Could you check a few things on this drawing? It's one solid part, dimensions in mm from its lowest x, y, z. A direction names the side the tool comes from. Round coordinates to 2 decimals unless told otherwise and drop trailing zeros. Write each loop counter-clockwise with the first axis right and the second up, starting at its lowest first coordinate (ties: lowest second). Pieces come first, ordered by that corner, then holes. Notation, with made-up numbers: (59, 42) -> (97, 42) arc R14 cw to (97, 69) -> close; hole circle Ø4 at (5.5, -7.75). An arc over 180 degrees is marked (long way). Answer in a Markdown table with one row per item. Add a question column.
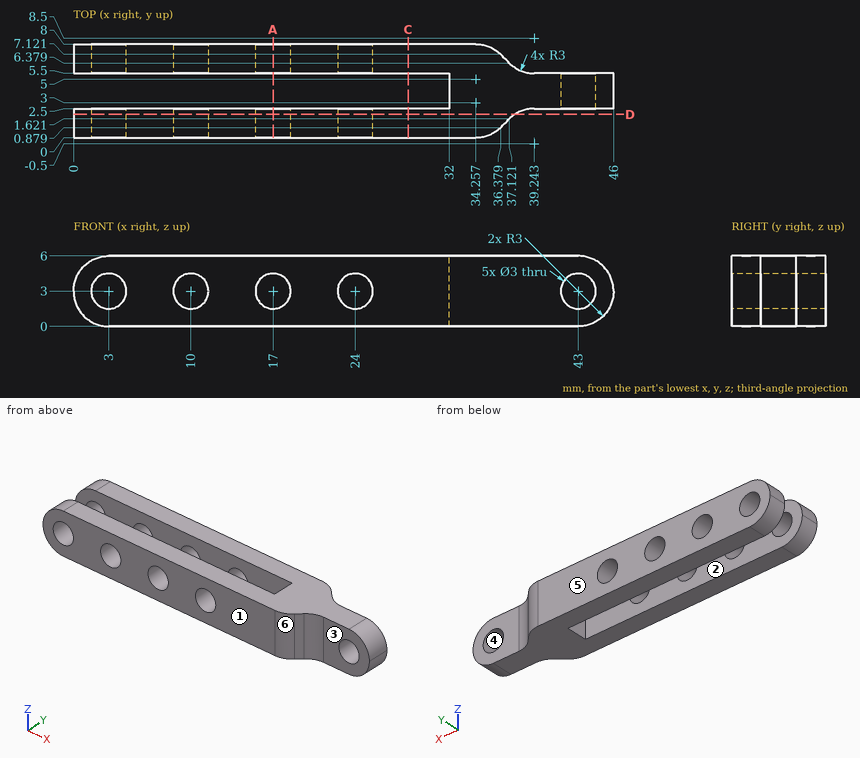
(1) Suppose I cut it at A-A, the plane x = 17. Please give me the cut outline in (y, z).
(2) Suppose I cut it at C-C, the plane x = 28.5. Please give me the cut outline in (y, z).
(3) For P1, Ø3, axis at x = 44.5, z = 3, coming from the -Y side; P2, Ø0.9, axis at y = 4, z = 3, coming from the -X side; P3, Ø1, axis at x = 41, z = 2, coming from the +Y side, each with a flat end and sliding along its axis, tell me the tip position at first contact or that it passes through.
(4) If we mould it in two halves opening along X, with no side actions, what happens to the marked faces 4, 5 and 6? For each: pulls with the +X half, pulls with the -X half, needs draft (parallel to the pull), parting line crosses it, or undercut.
(5) I need wall thicknesses on L1, parallel to Y at x = 2, z = 1; L2, parallel to Z at x = 24, y = 1.7; L3, parallel to X at y = 1.75, z = 2. Which ranges of each line are inside material? Lowest first, please.
(6) Suppose I cut it at D-D, the plane y = 2. State how many separate pieces and enclosed holes the cut face has, then the cut area to 3 significant figures.
(7) On a 3-axis mill with a long thin cutter (end or side, diameter ignored), from which of +Z, -Z, +X, -X, +Y, -Y can I reach the whole of each face in a straight line? I mean the marked faces 1, 2 and 3. Say none if no direction works.
Response:
| question | item | result |
|---|---|---|
| 1 | outline | (0, 0) -> (2.5, 0) -> (2.5, 1.5) -> (0, 1.5) -> close; (0, 4.5) -> (2.5, 4.5) -> (2.5, 6) -> (0, 6) -> close; (5.5, 0) -> (8, 0) -> (8, 1.5) -> (5.5, 1.5) -> close; (5.5, 4.5) -> (8, 4.5) -> (8, 6) -> (5.5, 6) -> close |
| 2 | outline | (0, 0) -> (2.5, 0) -> (2.5, 6) -> (0, 6) -> close; (5.5, 0) -> (8, 0) -> (8, 6) -> (5.5, 6) -> close |
| 3 | P1 | y = 2.5 |
| 3 | P2 | x = 32 |
| 3 | P3 | y = 5.5 |
| 4 | face 4 | undercut |
| 4 | face 5 | needs draft |
| 4 | face 6 | pulls with the +X half |
| 5 | L1 | 0 to 2.5, 5.5 to 8 |
| 5 | L2 | 0 to 1.5, 4.5 to 6 |
| 5 | L3 | 0.17 to 1.88, 4.12 to 8.88, 11.12 to 15.88, 18.12 to 22.88, 25.12 to 37.26 |
| 6 | separate pieces | 1 |
| 6 | enclosed holes | 4 |
| 6 | area | 193 mm² |
| 7 | face 1 | +Z, -Z, +X, -X, -Y |
| 7 | face 2 | +Z, -Z, -X |
| 7 | face 3 | +Z, -Z, +X, -Y |
